```python
from build123d import *

# Parameters (mm, degrees)
SKETCH1_W                      = 12.7
SKETCH1_H                      = 25
BOSS_EXTRUDE1_DEPTH            = 3
CUT_EXTRUDE1_DEPTH             = 26.967720347
CUT_EXTRUDE1_DEPTH_BACK        = 17.18
M3_CLEARANCE_HOLE1_D           = 3.4
M3_CLEARANCE_HOLE1_DEPTH       = 3
M3_CLEARANCE_HOLE1_CSINK_D     = 3.45
M3_CLEARANCE_HOLE1_CSINK_ANGLE = 90
M3_CLEARANCE_HOLE1_TIP         = 1.021463052


with BuildPart() as part:
    # Sketch1 → Boss-Extrude1 (new body)
    with BuildSketch(Plane(origin=(0, 0, 0), x_dir=(1, 0, 0), z_dir=(0, 1, 0))):
        Rectangle(SKETCH1_W, SKETCH1_H)
    extrude(amount=BOSS_EXTRUDE1_DEPTH)

    # Sketch2 → Cut-Extrude1 (cut, two sides: drawn at the far end of the back side and taken through both)
    with BuildSketch(Plane.XY.offset(12.5).offset(-CUT_EXTRUDE1_DEPTH_BACK)):
        with BuildLine():
            Line((-15.481656951, -23.428816816), (-1.7, 0))
            ThreePointArc((-1.7, 0), (0, 0.972308292), (1.7, 0))
            Line((1.7, 0), (15.481656951, -23.428816816))
            Line((15.481656951, -23.428816816), (15.481656951, -77.792169389))
            Line((15.481656951, -77.792169389), (-15.481656951, -77.792169389))
            Line((-15.481656951, -77.792169389), (-15.481656951, -23.428816816))
        make_face()
    extrude(amount=CUT_EXTRUDE1_DEPTH + CUT_EXTRUDE1_DEPTH_BACK, mode=Mode.SUBTRACT)

    # M3 Clearance Hole1
    with Locations(Plane(origin=(0, 3, 0), x_dir=(1, 0, 0), z_dir=(0, 1, 0))):
        with Locations((-4.025, 8.59), (4.025, 8.59)):
            CounterSinkHole(M3_CLEARANCE_HOLE1_D / 2, M3_CLEARANCE_HOLE1_CSINK_D / 2, depth=M3_CLEARANCE_HOLE1_DEPTH, counter_sink_angle=M3_CLEARANCE_HOLE1_CSINK_ANGLE)
            with Locations((0, 0, -(M3_CLEARANCE_HOLE1_DEPTH + M3_CLEARANCE_HOLE1_TIP / 2))):  # 118° drill point
                Cone(0, M3_CLEARANCE_HOLE1_D / 2, M3_CLEARANCE_HOLE1_TIP, mode=Mode.SUBTRACT)


solid = part.part
```
Here's how the part is built. I have some questions about the finished solid (model axes, mm). A direction names the side the tool comes from. Coordinates: 2 decimals unless noted, no trailing zeros. Write each loop counter-clockwise with the first axis right and the second up, starting at its lowest first coordinate (ties: lowest second). Pieces come first, ordered by that corner, then holes. Notation, with made-up numbers: (5, 15.5) - (9, 15.5) arc R25 ccw to (9, 39.5) - close; hole circle Ø2 at (35.25, 23). An arc over 180 degrees is marked (long way). One line per item, written item: value.
1) Suppose I cut it at B-B on y = 1.6. Write out the boundary of the cut face in (x, z) (3 decimals).
Model answer:
outline: (-6.35, -12.5) - (6.35, -12.5) - (6.35, 12.5) - (-6.35, 12.5) - close; hole circle Ø3.4 at (-4.025, -8.59); hole circle Ø3.4 at (4.025, -8.59)
2) Suppose I cut it at A-A on z = -8.59. Write out the boundary of the cut face in (x, y) (3 decimals), and give its area (3 significant figures).
Model answer:
outline: (-6.35, 0) - (-5.725, 0) - (-5.725, 2.975) - (-5.75, 3) - (-6.35, 3) - close; (-2.325, 0) - (2.325, 0) - (2.325, 2.975) - (2.3, 3) - (-2.3, 3) - (-2.325, 2.975) - close; (5.725, 0) - (6.35, 0) - (6.35, 3) - (5.75, 3) - (5.725, 2.975) - close
area: 17.7 mm²
3) I need wall thicknesses on line 1 along X through (y, z) = (1.7, -8.59) (3 decimals); line 2 along Z through (x, y) = (-0.25, 0.65); line 3 along X through (y, z) = (0.4, -9.5). Which ranges of each line are inside material? Lowest first, please.
Model answer:
line 1: x = -6.35 to -5.725, -2.325 to 2.325, 5.725 to 6.35
line 2: z = -12.5 to -4.68
line 3: x = -6.35 to -5.46, -2.59 to 2.59, 5.46 to 6.35
4) On a 3-axis mill with a long thin cutter (end or side, diameter ignored), from which of +Z, -Z, +X, -X, +Y, -Y can I reach the whole of each face in a straight line? I mean faces 1 (the cylindrical face through (-0.029, 0.972, 3.79)), 2 (the flat face through (6.35, 1, 0)). Say none if no direction works.
Model answer:
face 1: +Z, -Y
face 2: +Z, -Z, +X, +Y, -Y
5) Suppose I cut it at D-D on y = 0.35. Write out the boundary of the cut face in (x, z) (3 decimals).
Model answer:
outline: (-6.35, -12.5) - (6.35, -12.5) - (6.35, 12.5) - (1.438, 12.5) - (1.438, -4.68) - (-1.438, -4.68) - (-1.438, 12.5) - (-6.35, 12.5) - close; hole circle Ø3.4 at (-4.025, -8.59); hole circle Ø3.4 at (4.025, -8.59)
6) Suppose I cut it at C-C on z = 0.5. Write out the boundary of the cut face in (x, y), and give its area (3 significant figures).
Model answer:
outline: (-6.35, 0) - (-1.7, 0) arc R1.97 cw to (1.7, 0) - (6.35, 0) - (6.35, 3) - (-6.35, 3) - close
area: 35.8 mm²
7) I'm going to push a flat-ended pin straight in: P1, Ø2, axis at x = 4.025, z = -8.59, coming from the -Y side. Where does the tip first touch, or does it pass through?
Model answer:
P1: passes through
